```python
from build123d import *

# Parameters (mm, degrees)
F1_DEPTH = 12
F2_W     = 18
F2_H     = 150
F3_DEPTH = 120
F4_W     = 18
F4_H     = 150
F5_DEPTH = 18
F6_W     = 560
F6_H     = 150
F7_DEPTH = 12


with BuildPart() as f1:
    # F0 (on Top) → F1 (new body)
    with BuildSketch(Plane.XY):
        Polygon((-280, 0), (0, 0), (0, 257.8027844429), (-141.2238776684, 257.8027844429), (-141.2238776684, 334.6943855286), (-116.9423237443, 334.6943855286), (-170.564070344, 420), (-215.0802463293, 331.659168005), (-186.751767993, 331.659168005), (-186.751767993, 187.9933476448), (-231.2679439783, 187.9933476448), (-231.2679439783, 248.6972212791), (-320.3002810478, 248.6972212791), (-320.3002810478, 210), (-280, 210), align=None)
        Polygon((0, 257.8027844429), (0, 0), (280, 0), (280, 210), (320.3002810478, 210), (320.3002810478, 248.6972212791), (231.2679439783, 248.6972212791), (231.2679439783, 187.9933476448), (186.751767993, 187.9933476448), (186.751767993, 331.659168005), (215.0802463293, 331.659168005), (170.564070344, 420), (116.9423237443, 334.6943855286), (141.2238776684, 334.6943855286), (141.2238776684, 257.8027844429), align=None)
    extrude(amount=F1_DEPTH)

    # F2 (on face) → F3 (join)
    with BuildSketch(Plane.XY.offset(12)):
        with Locations((271, 75)):
            Rectangle(F2_W, F2_H)
        with Locations((-271, 75)):
            Rectangle(F2_W, F2_H)
    extrude(amount=F3_DEPTH)

    # F4 (on face) → F5 (join)
    with BuildSketch(Plane.XY.offset(132)):
        with Locations((-271, 75)):
            Rectangle(F4_W, F4_H)
        with BuildLine():
            Line((-262, 150), (-262, 0))
            Line((-262, 0), (280, 0))
            Line((280, 0), (280, 290.2253270149))
            ThreePointArc((280, 290.2253270149), (245.3046465179, 345.1352809089), (210.5378061533, 400))
            ThreePointArc((210.5378061533, 400), (185.6424554033, 363.2406210102), (154.8503190279, 331.2582075596))
            ThreePointArc((154.8503190279, 331.2582075596), (126.7121671615, 349.1136575609), (106.0016453266, 375.2220273018))
            ThreePointArc((106.0016453266, 375.2220273018), (82.2836881086, 339.6685760287), (48.3601950109, 313.6726915836))
            ThreePointArc((48.3601950109, 313.6726915836), (19.4703625217, 354.197972067), (0, 400))
            ThreePointArc((0, 400), (-33.0118277181, 338.4516060295), (-83.5312455893, 290.2253270149))
            ThreePointArc((-83.5312455893, 290.2253270149), (-152.6734230413, 334.7469853741), (-202.7220278978, 400))
            ThreePointArc((-202.7220278978, 400), (-239.2310011006, 334.5488326327), (-280, 271.6628313065))
            Line((-280, 271.6628313065), (-280, 150))
            Line((-280, 150), (-262, 150))
        make_face()
    extrude(amount=F5_DEPTH)

    # F6 (on face) → F7 (join)
    with BuildSketch(Plane.XZ):
        with Locations((0, 75)):
            Rectangle(F6_W, F6_H)
    extrude(amount=F7_DEPTH)


solid = f1.part
```
The listing builds one solid part. Answer for the finished solid, in the listing's coordinates (mm). A direction names the side the tool comes from. Coordinates: 2 decimals unless noted, no trailing zeros. Loops run counter-clockwise (first coordinate to the right, second up) from the corner with the lowest first, then second, coordinate; pieces in that order, holes last. Notation, with made-up numbers: M 47,47.5 L 62,47.5 A10 ccw 62,61.5 Z; hole C 25.5,34 d8. An arc over 180 degrees is marked long. Answer as CSV lines item,"result". Start each with the question number.
(1) Given pin 1 (9.5 mm diameter, centred on y = 291, z = 8.5, fed in from +X); pin 2 (13 mm diameter, centred on x = 3.5, z = 7, fed in from +Y); pin 3 (9.5 mm diameter, centred on x = 202, z = 9, fed in from +Y), each flat-ended and moving along its own axis, determine where each tip first touches the part or whether it passes through.
(2) The part is cut by section A-A (x = 202.5). Give the vertices of the cut face in (y, z).
(3) The part is cut by section C-C (z = 34). Give the vertices of the cut face in (x, y).
(4) For faces 4 (the flat face through (231.268, 219, 6)), 5 (the flat face through (201, 331.659, 6)), 6 (the flat face through (-300, 210, 6)), 7 (the flat face through (-201, 331.659, 6)), determine the directions among +Z, -Z, +X, -X, +Y, -Y from which every point of the face is accessible in a straight line to the end or side of a thin tool.
(5) The part is cut by section D-D (x = -273). Give the vertices of the cut face in (y, z).
(6) Find the intervals of material crossed by L1, parallel to Z at x = -78, y = 99; L2, parallel to X at y = 96, z = 49.5; L3, parallel to X at y = 328, z = 8, in increasing order. Write a range as [from, to].
(7) The mould has two halves that part along X. Classify faces 1 (the flat face through (-320.3, 230, 6)), 2 (the flat face through (-4, 158, 132)), 3 (the flat face through (276, 248.697, 6)): pulls with the +X half, pulls with the -X half, needs draft (parallel to the pull), parting line crosses it, or undercut.
(8) The part is cut by section B-B (y = 30). Give the vertices of the cut face in (x, z).
Determined:
1,pin 1,"x = 186.75"
1,pin 2,"y = 257.8"
1,pin 3,"y = 367.04"
2,outline,"M -12,0 L 187.99,0 L 187.99,12 L 0,12 L 0,132 L 386.59,132 L 386.59,150 L -12,150 Z; M 331.66,0 L 356.62,0 L 356.62,12 L 331.66,12 Z"
3,outline,"M -280,-12 L 280,-12 L 280,150 L 262,150 L 262,0 L -262,0 L -262,150 L -280,150 Z"
4,face 4,"-Z, +Y"
4,face 5,"-Z, +X"
4,face 6,"+Z, -Z, -X, -Y"
4,face 7,"-Z, -X"
5,outline,"M -12,0 L 248.7,0 L 248.7,12 L 150,12 L 150,132 L 281.83,132 L 281.83,150 L -12,150 Z"
6,L1,"[0, 12], [132, 150]"
6,L2,"[-280, -262], [262, 280]"
6,L3,"[-186.75, -141.22], [141.22, 186.75]"
7,face 1,"pulls with the -X half"
7,face 2,"undercut"
7,face 3,"needs draft"
8,outline,"M -280,0 L 280,0 L 280,150 L -280,150 Z; hole M -262,12 L 262,12 L 262,132 L -262,132 Z"
